Can you work these out from the drawing? Everything is in mm from the part's minimum corner. Give positions to 0.01 mm unless a question says otherwise; leave off trailing zeros. Order: outer loops, then holes, each group sorted by start corner. A loop starts at its lowest first (then second) coordinate and runs counter-clockwise, first axis right, second up. Notation, with made-up numbers: M -5,43 L 4,43 A19 cw 4,52 Z; hole C 48,50.5 d7. An arc over 180 degrees is marked long. Use a Markdown table: item, result. Add a question column.
Item 1: Suppose I cut it at C-C on x = 101.5. Write out the boundary of the cut face in (y, z).
Item 2: I'm going to push flat-ended pins straight in: pin 1 Ø6 at (x, z) = (88, 34) entering from -Y; pin 2 Ø5 at (y, z) = (7, 48.5) entering from -X; pin 3 Ø5 at (x, y) = (466.5, 4) entering from +Z. Where does each tip first touch, or does it pass through?
Item 3: Suppose I cut it at B-B on y = 4.5. Write out the boundary of the cut face in (x, z).
Item 4: If I drill on L1, parallel to X at y = 8.25, z = 44.5; L2, parallel to Z at x = 343, y = 2, over which ranges is the centre line in solid material (lowest first)? Write a range as from..to.
Item 5: Suppose I cut it at A-A on z = 54.5. Write out the boundary of the cut face in (x, y).
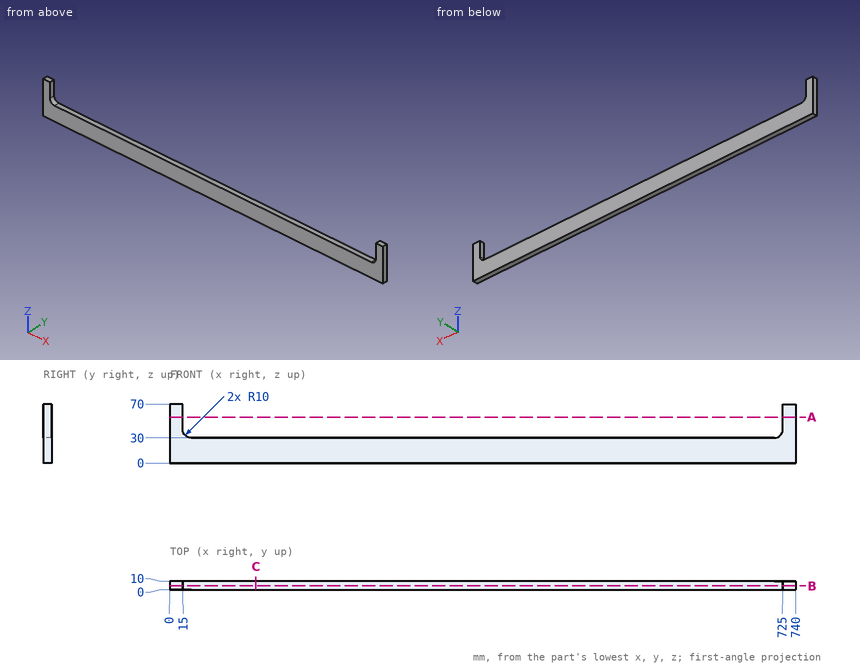
Findings below:
| question | item | result |
|---|---|---|
| 1 | outline | M 0,0 L 10,0 L 10,30 L 0,30 Z |
| 2 | pin 1 | passes through |
| 2 | pin 2 | stops at x = 0 |
| 2 | pin 3 | stops at z = 30 |
| 3 | outline | M 0,0 L 740,0 L 740,70 L 725,70 L 725,40 A10 cw 715,30 L 25,30 A10 cw 15,40 L 15,70 L 0,70 Z |
| 4 | L1 | x = 0..15, 725..740 |
| 4 | L2 | z = 0..30 |
| 5 | outline | M 0,0 L 15,0 L 15,10 L 0,10 Z; M 725,0 L 740,0 L 740,10 L 725,10 Z |
